Part model, mm, in its own coordinate system. Face numbers are marked on the shaded views. A direction names the side the tool comes from. Round coordinates to 2 decimals unless told otherwise and drop trailing zeros. Write each loop counter-clockwise with the first axis right and the second up, starting at its lowest first coordinate (ties: lowest second). Pieces come first, ordered by that corner, then holes. Notation, with made-up numbers: M 31,-16 L 80,-16 A6 ccw 80,-7 Z; hole C 84,85.25 d6. An arc over 180 degrees is marked long. One line per question, with ' | ' between items. Start each with the question number.
1) Saw through at A-A (y = 357). List the corners of the cut face in (x, z) (3 decimals).
2) Wall check: probe 1 along Z at (x, y) = (-1, 641); probe 2 along Z at (x, y) = (21.5, 297); probe 3 along X at (y, z) = (550.5, 25). Give the ranges that are in metal, low to high. Write a range as [from, to].
3) Tool access for the marked faces 1 and 2: list every direction of +Z, -Z, +X, -X, +Y, -Y with a clear straight run to the whole face (end or side of a thin tool).
4) Drop flat-ended pins along their axis: pin 1 Ø8 at (y, z) = (788, -19.5) entering from -X; pin 2 Ø3 at (x, y) = (-20, 804) entering from -Z; pin 3 Ø12 at (y, z) = (528.5, -13) entering from -X. Give the stop position or say it passes through.
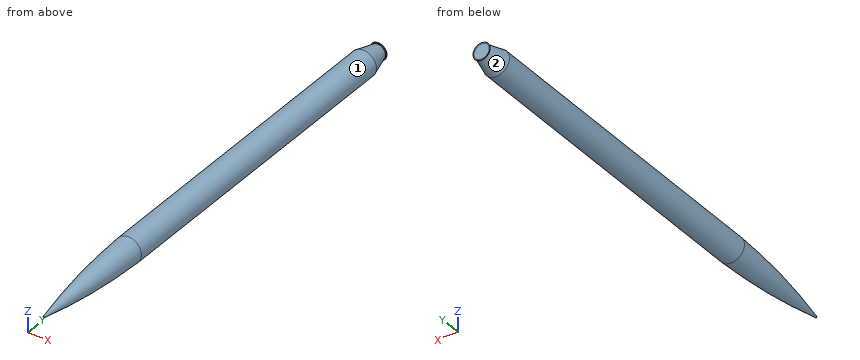
```python
from build123d import *


with BuildPart() as part:
    # Sketch2 → Revolve1 (revolve)
    with BuildSketch(Plane.XY, mode=Mode.PRIVATE) as revolve1_sk:
        with BuildLine():
            Line((0, 947.42), (0, 6.753760064))
            ThreePointArc((0, 6.753760064), (1.004358981, 7.115605787), (1.547169826, 8.034858568))
            ThreePointArc((1.547169826, 8.034858568), (20.581846727, 138.066176315), (28.575, 269.24))
            Line((28.575, 269.24), (28.575, 947.42))
            Line((28.575, 947.42), (0, 947.42))
        make_face()
    revolve(revolve1_sk.sketch.rotate(Axis((0, 0, 0), (0, 1, 0)), 90), axis=Axis((0, 0, 0), (0, 1, 0)))

    # Sketch3 → Revolve2 (revolve)
    with BuildSketch(Plane.XY):
        with BuildLine():
            Line((-28.575, 994.156), (-28.575, 947.42))
            Line((-28.575, 947.42), (0, 947.42))
            Line((0, 947.42), (0, 1040.13))
            Line((0, 1040.13), (-16.6116, 1040.13))
            Line((-16.6116, 1040.13), (-18.669, 1040.681278669))
            Line((-18.669, 1040.681278669), (-18.872794116, 1039.920708673))
            Line((-18.872794116, 1039.920708673), (-17.219933754, 1039.477826074))
            ThreePointArc((-17.219933754, 1039.477826074), (-16.757242508, 1039.122790594), (-16.681118386, 1038.544570482))
            Line((-16.681118386, 1038.544570482), (-28.575, 994.156))
        make_face()
    revolve(axis=Axis((0, 1040.13, 0), (0, -1, 0)))


solid = part.part
```
Answer key:
1) outline: C 0,0 d57.15
2) probe 1: z = [-28.56, 28.56] | probe 2: z = [-18.82, 18.82] | probe 3: x = [-13.84, 13.84]
3) face 1: +Y, -Y | face 2: none
4) pin 1: stops at x = -24.01 | pin 2: stops at z = -21.78 | pin 3: stops at x = -27.7
